Input: part model. Units: mm. Frame: model coordinates. A direction names the side the tool comes from. Round coordinates to 2 decimals unless told otherwise and drop trailing zeros. Order: outer loops, then holes, each group sorted by start corner. A loop starts at its lowest first (then second) coordinate and runs counter-clockwise, first axis right, second up. Notation, with made-up numbers: (-19.75, 63) -> (5.25, 63) arc R26 cw to (5.25, 94) -> close; hole circle Ø7 at (62, -34.5). An arc over 180 degrees is marked (long way). Answer as CSV lines item,"result". Start each with the question number.
1) Section query D-D, the plane y = 22.5. Output: boundary loops of the cut face in (x, z).
2) Mould query, pull axis X, two halves, no side actions, for faces 5 (the face through (28, 15, 54)), 6 (the face through (0, -27, 10.875)), 7 (the face through (29, 25, 8.5)), 8 (the face through (21.4, -19.14, 37.93)). Classes: +X half, -X half, draft (parallel to the pull), parting line (faces both ways), or undercut.
3) Section query B-B, the plane x = -15. Output: boundary loops of the cut face in (y, z) (3 decimals).
4) Section query A-A, the plane z = 9.5. Output: boundary loops of the cut face in (x, y), and give its area (3 significant figures).
5) First-contact query: P1, Ø2, axis at x = -20, y = 13.5, coming from the +Z side; P2, Ø17, axis at y = -5.5, z = 37, coming from the +X side; P3, Ø2, axis at x = -27, z = 13, coming from the -Y side; P4, Ø1.8, axis at x = 22.5, z = 16.5, coming from the -Y side. Flat tips, straight axial feed; report the tip coordinate or a pass-through.
6) Line query: L1, parallel to Z at x = -29.7, y = 15; L2, parallel to Y at x = 2.5, z = 19; L3, parallel to Z at x = -22.95, y = 0. Output: solid intervals per line, ascending.
7) Access query for faces 1 (the face through (22.97, 28.04, 22.77)), 2 (the face through (-2.4, -20.3, 6.5)), 3 (the face through (21.44, 19.1, 37.93)), 4 (the face through (0, 32, 8.5)). Directions: +Z, -Z, +X, -X, +Y, -Y. A direction counts if a zero-diameter tool reaches every point of the face in a straight line with its end or side. Return the directions, or none.
```python
from build123d import *

# Parameters (mm, degrees)
F1_R      = 35.5
F2_DEPTH  = 8.5
F0_R      = 30.25
F3_DEPTH  = 8.5
F5_W      = 68
F5_H      = 30.5
F6_DEPTH  = 60
F7_R      = 35.25
F8_DEPTH  = 2
F9_DEPTH  = 100
F10_R     = 19
F11_DEPTH = 12
F12_R     = 26.1
F13_DEPTH = 9.5
F15_DEPTH = 6.5
F17_DEPTH = 25
F18_R     = 12.84
F19_DEPTH = 10.7
F20_R     = 10.8
F21_DEPTH = 25
F22_R     = 12.84
F23_DEPTH = 9.5
F24_R     = 0.8
F25_DEPTH = 3
F26_R     = 2.55
F27_DEPTH = 5
F28_R     = 10.8
F29_DEPTH = 25
F30_R     = 12.84
F31_DEPTH = 10.7
F32_R     = 1.13
F33_DEPTH = 6
F34_R     = 1.13
F35_DEPTH = 6


with BuildPart() as f2:
    # F1 (on Top) → F2 (new body)
    with BuildSketch(Plane.XY):
        Circle(F1_R)
    extrude(amount=F2_DEPTH)

    # F0 (on Top) → F3 (cut)
    with BuildSketch(Plane.XY):
        Circle(F0_R)
    extrude(amount=F3_DEPTH, mode=Mode.SUBTRACT)

    # F5 (on face) → F6 (join)
    with BuildSketch(Plane.XY.offset(8.5)):
        with Locations((0, 15.25)):
            Rectangle(F5_W, F5_H)
        with Locations((0, -15.25)):
            Rectangle(F5_W, F5_H)
    extrude(amount=F6_DEPTH)

    # F7 (on face) → F8 (join)
    with BuildSketch(Plane(origin=(0, 0, 8.5), x_dir=(1, 0, 0), z_dir=(0, 0, -1))):
        Circle(F7_R)
    extrude(amount=F8_DEPTH)

    # F4 (on face) → F9 (cut, symmetric)
    with BuildSketch(Plane.XY.offset(8.5)):
        with BuildLine():
            Line((-19.3, -20), (19.3, -20))
            ThreePointArc((19.3, -20), (21.4213203436, -19.1213203436), (22.3, -17))
            Line((22.3, -17), (22.3, 17))
            ThreePointArc((22.3, 17), (21.4213203436, 19.1213203436), (19.3, 20))
            Line((19.3, 20), (-19.3, 20))
            ThreePointArc((-19.3, 20), (-21.4213203436, 19.1213203436), (-22.3, 17))
            Line((-22.3, 17), (-22.3, -17))
            ThreePointArc((-22.3, -17), (-21.4213203436, -19.1213203436), (-19.3, -20))
        make_face()
    extrude(amount=F9_DEPTH, both=True, mode=Mode.SUBTRACT)

    # F10 (on face) → F11 (cut)
    with BuildSketch(Plane.XZ.offset(30.5)):
        with Locations((0, 38.5)):
            Circle(F10_R)
    extrude(amount=-F11_DEPTH, mode=Mode.SUBTRACT)

    # F12 (on face) → F13 (cut)
    with BuildSketch(Plane.XZ.offset(30.5)):
        with Locations((0, 38.5)):
            Circle(F12_R)
    extrude(amount=-F13_DEPTH, mode=Mode.SUBTRACT)

    # F14 (on face) → F15 (cut)
    with BuildSketch(Plane.XZ.offset(30.5)):
        with BuildLine():
            Line((-24.625, 10.875), (24.625, 10.875))
            ThreePointArc((24.625, 10.875), (26.7463203436, 11.7536796564), (27.625, 13.875))
            Line((27.625, 13.875), (27.625, 63.125))
            ThreePointArc((27.625, 63.125), (26.7463203436, 65.2463203436), (24.625, 66.125))
            Line((24.625, 66.125), (-24.625, 66.125))
            ThreePointArc((-24.625, 66.125), (-26.7463203436, 65.2463203436), (-27.625, 63.125))
            Line((-27.625, 63.125), (-27.625, 13.875))
            ThreePointArc((-27.625, 13.875), (-26.7463203436, 11.7536796564), (-24.625, 10.875))
        make_face()
    extrude(amount=-F15_DEPTH, mode=Mode.SUBTRACT)

    # F16 (on face) → F17 (cut)
    with BuildSketch(Plane(origin=(-34, 0, 0), x_dir=(0, -1, 0), z_dir=(-1, 0, 0))):
        with BuildLine():
            ThreePointArc((0, 27.7), (7.6367532368, 30.8632467632), (10.8, 38.5))
            ThreePointArc((10.8, 38.5), (-7.6367532368, 46.1367532368), (0, 27.7))
        make_face()
    extrude(amount=-F17_DEPTH, mode=Mode.SUBTRACT)

    # F18 (on face) → F19 (cut)
    with BuildSketch(Plane(origin=(-34, 0, 0), x_dir=(0, -1, 0), z_dir=(-1, 0, 0))):
        with Locations((0, 38.5)):
            Circle(F18_R)
    extrude(amount=-F19_DEPTH, mode=Mode.SUBTRACT)

    # F20 (on face) → F21 (cut)
    with BuildSketch(Plane(origin=(0, 30.5, 0), x_dir=(-1, 0, 0), z_dir=(0, 1, 0))):
        with Locations((0, 38.5)):
            Circle(F20_R)
    extrude(amount=-F21_DEPTH, mode=Mode.SUBTRACT)

    # F22 (on face) → F23 (cut)
    with BuildSketch(Plane(origin=(0, 30.5, 0), x_dir=(-1, 0, 0), z_dir=(0, 1, 0))):
        with Locations((0, 38.5)):
            Circle(F22_R)
    extrude(amount=-F23_DEPTH, mode=Mode.SUBTRACT)

    # F24 (on face) → F25 (cut)
    with BuildSketch(Plane.XZ.offset(24)):
        with Locations((-22, 60.5)):
            Circle(F24_R)
        with Locations((22, 60.5)):
            Circle(F24_R)
        with Locations((22, 16.5)):
            Circle(F24_R)
        with Locations((-22, 16.5)):
            Circle(F24_R)
    extrude(amount=-F25_DEPTH, mode=Mode.SUBTRACT)

    # F26 (on face) → F27 (cut)
    with BuildSketch(Plane(origin=(0, 30.5, 0), x_dir=(-1, 0, 0), z_dir=(0, 1, 0))):
        with Locations((-25.4, 55)):
            Circle(F26_R)
        with Locations((25.4, 55)):
            Circle(F26_R)
        with Locations((25.4, 22)):
            Circle(F26_R)
        with Locations((-25.4, 22)):
            Circle(F26_R)
    extrude(amount=-F27_DEPTH, mode=Mode.SUBTRACT)

    # F28 (on face) → F29 (cut)
    with BuildSketch(Plane.YZ.offset(34)):
        with Locations((0, 38.5)):
            Circle(F28_R)
    extrude(amount=-F29_DEPTH, mode=Mode.SUBTRACT)

    # F30 (on face) → F31 (cut)
    with BuildSketch(Plane.YZ.offset(34)):
        with Locations((0, 38.5)):
            Circle(F30_R)
    extrude(amount=-F31_DEPTH, mode=Mode.SUBTRACT)

    # F32 (on face) → F33 (cut)
    with BuildSketch(Plane.YZ.offset(34)):
        with Locations((-15, 53.5)):
            Circle(F32_R)
        with Locations((15, 53.5)):
            Circle(F32_R)
        with Locations((15, 23.5)):
            Circle(F32_R)
        with Locations((-15, 23.5)):
            Circle(F32_R)
    extrude(amount=-F33_DEPTH, mode=Mode.SUBTRACT)

    # F34 (on face) → F35 (cut)
    with BuildSketch(Plane(origin=(-34, 0, 0), x_dir=(0, -1, 0), z_dir=(-1, 0, 0))):
        with Locations((-15, 23.5)):
            Circle(F34_R)
        with Locations((15, 23.5)):
            Circle(F34_R)
        with Locations((15, 53.5)):
            Circle(F34_R)
        with Locations((-15, 53.5)):
            Circle(F34_R)
    extrude(amount=-F35_DEPTH, mode=Mode.SUBTRACT)


solid = f2.part
```
Findings:
1,outline,"(-34, 8.5) -> (-27.46, 8.5) -> (-27.46, 0) -> (-20.22, 0) -> (-20.22, 6.5) -> (20.22, 6.5) -> (20.22, 0) -> (27.46, 0) -> (27.46, 8.5) -> (34, 8.5) -> (34, 68.5) -> (-34, 68.5) -> close; hole circle Ø25.68 at (0, 38.5)"
2,face 5,"+X half"
2,face 6,"undercut"
2,face 7,"draft"
2,face 8,"undercut"
3,outline,"(-32.175, 0) -> (-26.269, 0) -> (-26.269, 6.5) -> (-20, 6.5) -> (-20, 26.838) -> (-21, 26.838) -> (-21, 17.141) -> (-24, 17.141) -> (-24, 10.875) -> (-30.5, 10.875) -> (-30.5, 8.5) -> (-32.175, 8.5) -> close; (-30.5, 66.125) -> (-24, 66.125) -> (-24, 59.859) -> (-21, 59.859) -> (-21, 50.162) -> (-20, 50.162) -> (-20, 68.5) -> (-30.5, 68.5) -> close; (20, 6.5) -> (26.269, 6.5) -> (26.269, 0) -> (32.175, 0) -> (32.175, 8.5) -> (30.5, 8.5) -> (30.5, 68.5) -> (20, 68.5) -> close"
4,outline,"(-34, -30.5) -> (34, -30.5) -> (34, 30.5) -> (-34, 30.5) -> close; hole (-22.3, -17) arc R3 ccw to (-19.3, -20) -> (19.3, -20) arc R3 ccw to (22.3, -17) -> (22.3, 17) arc R3 ccw to (19.3, 20) -> (-19.3, 20) arc R3 ccw to (-22.3, 17) -> close"
4,area,"2,370 mm^2"
5,P1,"passes through"
5,P2,"stops at x = 34"
5,P3,"stops at y = -30.5"
5,P4,"stops at y = -24"
6,L1,"z = 0 to 22.37, 24.63 to 52.37, 54.63 to 68.5"
6,L2,"y = -21 to -20, 20 to 30.5"
6,L3,"z = 6.5 to 27.7, 49.3 to 68.5"
7,face 1,"+Y"
7,face 2,"-Z"
7,face 3,"+Z, -Z"
7,face 4,"+Z, +X, -X, +Y"
